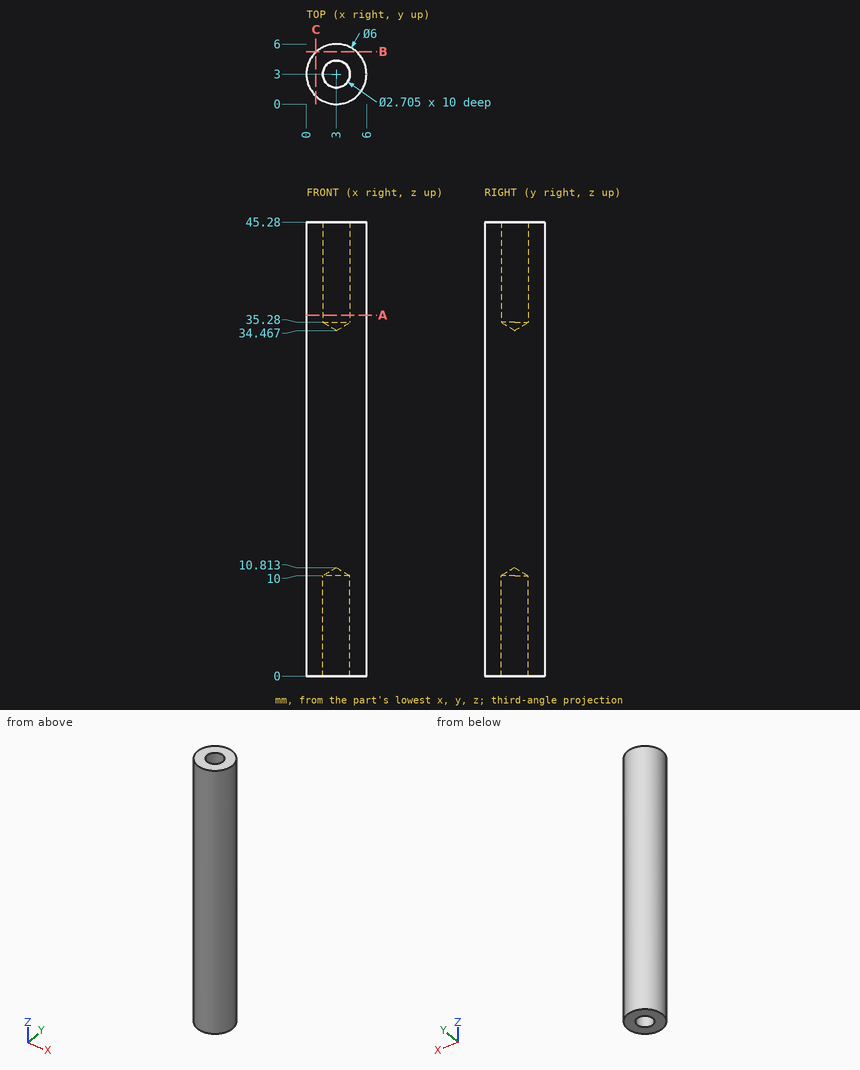
Design review of the part shown in the three views and the two pictorial views. Dimensions are in mm from the part's minimum x, y and z. Give positions to 0.01 mm unless a question says otherwise; leave off trailing zeros. Loops run counter-clockwise (first coordinate to the right, second up) from the corner with the lowest first, then second, coordinate; pieces in that order, holes last. Notation, with made-up numbers: (25, 74) -> (42, 74) arc R27 ccw to (42, 105) -> close; hole circle Ø10 at (38, 68.25). An arc over 180 degrees is marked (long way). Write each question's results on one line, items separated by ' | '.
Q1. Take a section at C-C, the plane x = 0.95. Write out the cut boundary in (y, z).
Reply:
outline: (0.81, 0) -> (5.19, 0) -> (5.19, 45.28) -> (0.81, 45.28) -> close
Q2. Take a section at B-B, the plane y = 5.25. Write out the cut boundary in (x, z).
Reply:
outline: (1.02, 0) -> (4.98, 0) -> (4.98, 45.28) -> (1.02, 45.28) -> close
Q3. For pin 1 Ø1.5 at (x, z) = (2.5, 16.5) entering from -Y; pin 2 Ø1.5 at (x, z) = (0.5, 9) entering from +Y; pin 3 Ø1.5 at (y, z) = (1, 17.5) entering from +X, all flat-tipped, find the tip position at first contact; note any pin that passes through.
Reply:
pin 1: stops at y = 0 | pin 2: stops at y = 5.44 | pin 3: stops at x = 5.73
Q4. Wall thickness on L1, parallel to Y at x = 3, z = 7.25; L2, parallel to X at y = 3.15, z = 36.5; L3, parallel to Y at x = 3.7, z = 39.5: over which ranges is each line inside the solid? List them lowest first.
Reply:
L1: y = 0 to 1.65, 4.35 to 6 | L2: x = 0 to 1.66, 4.34 to 6 | L3: y = 0.08 to 1.84, 4.16 to 5.92
Q5. Take a section at A-A, the plane z = 36. Write out the cut boundary in (x, y) (1 decimal), plus the area to 3 significant figures.
Reply:
outline: circle Ø6 at (3, 3); hole circle Ø2.7 at (3, 3) | area: 22.5 mm²
